Job drawing, mm, ordinate dimensions from the low corner. One solid piece. A direction names the side the tool comes from. Round coordinates to 2 decimals unless told otherwise and drop trailing zeros. Loops run counter-clockwise (first coordinate to the right, second up) from the corner with the lowest first, then second, coordinate; pieces in that order, holes last. Notation, with made-up numbers: M 87.25,6 L 120.25,6 A23 ccw 120.25,18 Z; hole C 59.25,69 d1. An arc over 180 degrees is marked long. Put each result on its own line as item: value. Start each with the question number.
1) Slice it at B-B on z = 2.15. Give the cut face in (x, y) (1 decimal).
2) Drop flat-ended pins along their axis: pin 1 Ø6 at (x, y) = (12, 7.5) entering from +Z; pin 2 Ø1.5 at (y, z) = (2.5, 1) entering from +X. Give the stop position or say it passes through.
3) Which spindle directions (+Z, -Z, +X, -X, +Y, -Y) get a long thin tool onto all of the face, cutting with end or side? Do the marked faces 1 and 2. Say none if no direction does.
4) Slice it at C-C on y = 2.75. Give the cut face in (x, z).
5) Pull direction Y, two halves, no side cores. Call the marked faces 3, 4, 5 and 6: +Y half, -Y half, draft (parallel to the pull), parting line (faces both ways), or undercut.
6) Slice it at D-D on y = 7.5. Give the cut face in (x, z).
7) Slice it at A-A on x = 3. Give the cut face in (y, z).
8) Probe line 1 along Y through (x, z) = (7, 2.4) (1 decimal); line 2 along Y through (x, z) = (6, 0.8) (1 decimal); line 3 along X through (y, z) = (9.25, 0.45) (1 decimal). List the from-to ranges inside material, lowest first.
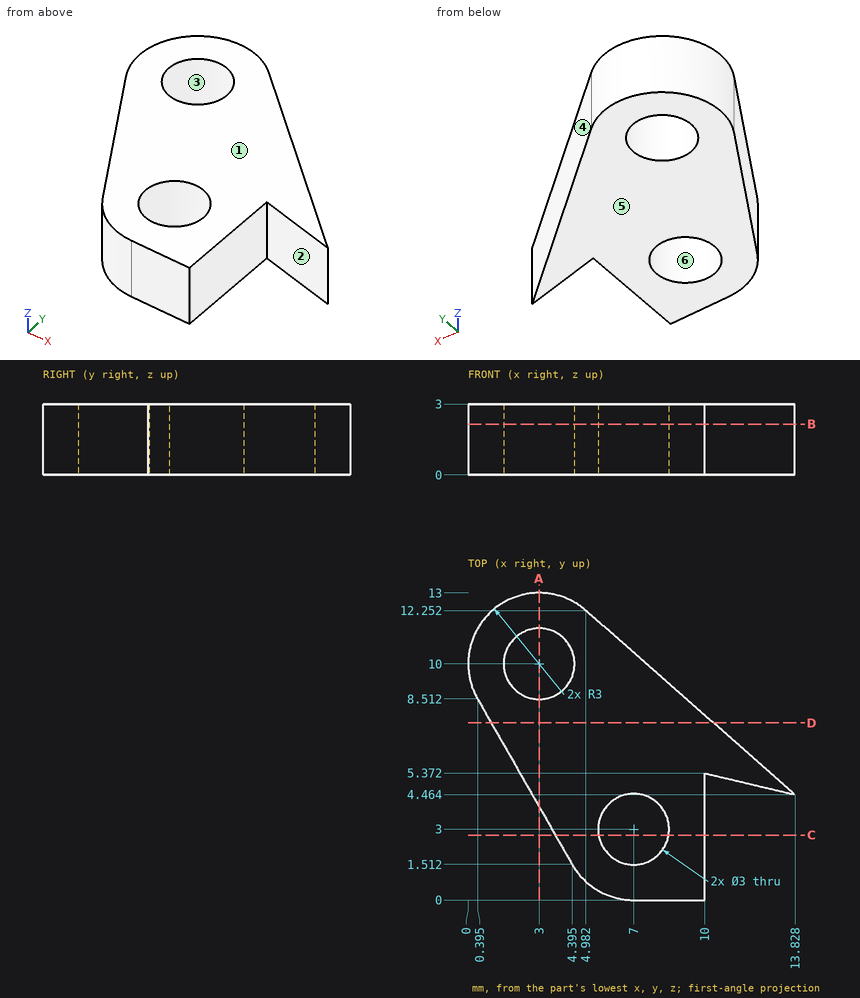
Recorded:
1. outline: M 0.4,8.5 L 4.4,1.5 A3 ccw 7,0 L 10,0 L 10,5.4 L 13.8,4.5 L 5,12.3 A3 ccw Z; hole C 3,10 d3; hole C 7,3 d3
2. pin 1: stops at z = 3
2. pin 2: stops at x = 10
3. face 1: +Z, +X, -X, +Y, -Y
3. face 2: +Z, -Z, -Y
4. outline: M 3.69,0 L 5.52,0 L 5.52,3 L 3.69,3 Z; M 8.48,0 L 10,0 L 10,3 L 8.48,3 Z
5. face 3: undercut
5. face 4: +Y half
5. face 5: draft
5. face 6: undercut
6. outline: M 0.97,0 L 10.38,0 L 10.38,3 L 0.97,3 Z
7. outline: M 3.95,0 L 8.5,0 L 8.5,3 L 3.95,3 Z; M 11.5,0 L 13,0 L 13,3 L 11.5,3 Z
8. line 1: y = 0 to 1.5, 4.5 to 10.5
8. line 2: y = 0.2 to 1.9, 4.1 to 11.4
8. line 3: x = 0.1 to 1.7, 4.3 to 8.4
